Answer from the drawing. Dimensions are ordinates in mm from the lowest x, y and z of the part. A direction names the side the tool comes from. Coordinates: 2 decimals unless noted, no trailing zeros. Order: outer loops, then holes, each group sorted by start corner. A loop starts at its lowest first (then second) coordinate and runs counter-clockwise, first axis right, second up. Notation, with made-up numbers: (-2, 2) - (47, 2) arc R7 cw to (47, 14) - close; hole circle Ø10 at (-10.5, 77). An arc over 180 degrees is marked (long way). Use CSV: the item, a comma, the result in double quotes. Start each with the question number.
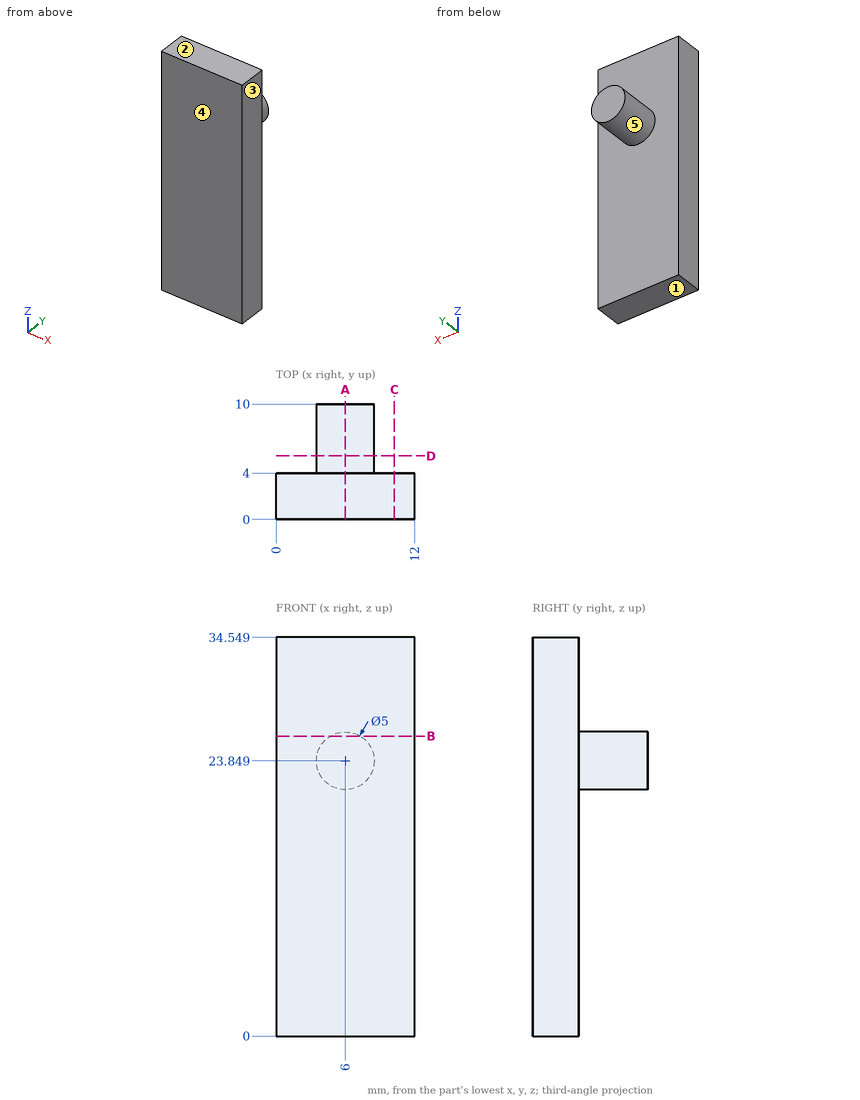
1) The part is cut by section A-A on x = 6. Determine the outline of the cut face in (y, z).
2) The part is cut by section B-B on z = 26. Determine the outline of the cut face in (x, y).
3) The part is cut by section C-C on x = 10.25. Determine the outline of the cut face in (y, z).
4) For a pull along Z with two mould halves and no side action, classify the marked faces 1, 2 and 3 as +Z half, -Z half, draft (parallel to the pull), parting line (faces both ways), or undercut.
5) For the marked faces 4 and 5, determine the directions among +Z, -Z, +X, -X, +Y, -Y from which every point of the face is accessible in a straight line to the end or side of a thin tool.
6) Straight lines are drawn through the part: line 1 (Y direction, x = 11.5, z = 9.5); line 2 (Z direction, x = 6, y = 6.25); line 3 (Z direction, x = 6.5, y = 7). For each, find the intervals that lie inside material, in ascending order. Write a range as [from, to].
7) The part is cut by section D-D on y = 5.5. Determine the outline of the cut face in (x, z), plus the area to 3 significant figures.
8) Flat-ended cylindrical pins translate along their axes: P1, Ø5, axis at y = 8, z = 10.5, coming from the -X side (1 decimal); P2, Ø5, axis at x = 7.5, y = 1, coming from the -Z side; P3, Ø1.5, axis at x = 8, y = 7, coming from the -Z side. Find the tip coordinate at first contact, or state that the pin passes through.
Answer key:
1,outline,"(0, 0) - (4, 0) - (4, 21.35) - (10, 21.35) - (10, 26.35) - (4, 26.35) - (4, 34.55) - (0, 34.55) - close"
2,outline,"(0, 0) - (12, 0) - (12, 4) - (7.27, 4) - (7.27, 10) - (4.73, 10) - (4.73, 4) - (0, 4) - close"
3,outline,"(0, 0) - (4, 0) - (4, 34.55) - (0, 34.55) - close"
4,face 1,"-Z half"
4,face 2,"+Z half"
4,face 3,"draft"
5,face 4,"+Z, -Z, +X, -X, -Y"
5,face 5,"+Y"
6,line 1,"[0, 4]"
6,line 2,"[21.35, 26.35]"
6,line 3,"[21.4, 26.3]"
7,outline,"circle Ø5 at (6, 23.85)"
7,area,"19.6 mm^2"
8,P1,"through"
8,P2,"z = 0"
8,P3,"z = 21.68"
